from build123d import *

# Parameters (mm, degrees)
SKETCH1_W           = 482.6
SKETCH1_H           = 50.8
BOSS_EXTRUDE1_DEPTH = 19.05
SKETCH5_W           = 508
SKETCH5_H           = 50.8
CUT_EXTRUDE1_DEPTH  = 246.940876462


with BuildPart() as part:
    # Sketch1 → Boss-Extrude1 (new body)
    with BuildSketch(Plane(origin=(0, 0, 0), x_dir=(1, 0, 0), z_dir=(0, 1, 0))):
        Rectangle(SKETCH1_W, SKETCH1_H)
    extrude(amount=BOSS_EXTRUDE1_DEPTH)

    # Sketch5 → Cut-Extrude1 (cut, through all)
    with BuildSketch(Plane(origin=(-0.481532302, 2.873320636, 16.634752254), x_dir=(0.9995934063300581, 0.0049512943147540294, 0.028080361573174478), z_dir=(-0.028513367553161754, 0.17014029390333138, 0.9850072427455884))):
        with Locations((0, 9.697527332)):
            Rectangle(SKETCH5_W, SKETCH5_H)
    cut_extrude1 = extrude(amount=CUT_EXTRUDE1_DEPTH, mode=Mode.SUBTRACT)

    # Mirror1: Cut-Extrude1 across plane
    add(cut_extrude1.mirror(Plane.XY), mode=Mode.SUBTRACT)


solid = part.part
Geometry: final body of the model. Coordinates: model frame, mm. Coordinates: 2 decimals unless noted, no trailing zeros. Order: outer loops, then holes, each group sorted by start corner. A loop starts at its lowest first (then second) coordinate and runs counter-clockwise, first axis right, second up.
(1) Section query B-B (x = -170.5). Return the cut outline in (y, z).
(2) First-contact query: pin 1 (1.5 mm diameter, centred on x = 22.5, y = 2.5, fed in from -Z); pin 2 (2 mm diameter, centred on x = 162, y = 11, fed in from +Z). Flat tips, straight axial feed; report the tip coordinate or a pass-through.
(3) Material intervals for probe 1 along Z at (x, y) = (-209, 5.75); probe 2 along Z at (x, y) = (-22.5, 4.5), sorted ascending.
(4) Section query A-A (y = 5). Return the cut outline in (x, z), plus the area to 3 significant figures.
Solution:
1. outline: (0, -12.21) - (19.05, -8.92) - (19.05, 8.92) - (0, 12.21) - close
2. pin 1: stops at z = -17.5
2. pin 2: stops at z = 20.11
3. probe 1: z = -10.1 to 10.1
3. probe 2: z = -15.72 to 15.72
4. outline: (-241.3, -9.3) - (241.3, -23.27) - (241.3, 23.27) - (-241.3, 9.3) - close
4. area: 15,700 mm2
